Print and shaded views of the part. All mm, measured from the part's lowest x, y and z. A direction names the side the tool comes from. Give positions to 0.01 mm unless a question says otherwise; leave off trailing zeros. Write each loop counter-clockwise with the first axis right and the second up, starting at its lowest first coordinate (ties: lowest second). Pieces come first, ordered by that corner, then holes. Notation, with made-up numbers: M 21.5,27.5 L 55.5,27.5 A22 ccw 55.5,47.5 Z; hole C -10,41 d7. An arc over 180 degrees is marked long. One line per question, with ' | ' between items. Start each with the question number.
1. Wall check: L1, parallel to X at y = 2.8, z = 6.7 (3 decimals); L2, parallel to X at y = 6.75, z = 4.25; L3, parallel to Y at x = 12.5, z = 8. Give the ranges that are in metal, low to high.
2. Cut at C-C, the plane x = 10.25. Write the cut outline in (y, z), then the cut area to 3 significant figures.
3. Which spindle directions (+Z, -Z, +X, -X, +Y, -Y) get a long thin tool onto all of the face, cutting with end or side? Do the marked faces 1 and 2. Say none if no direction does.
4. Pull direction X, two halves, no side cores. Call the marked faces 3, 4, 5 and 6: released by +X, released by -X, zero draft, split by the parting line, or undercut.
5. Cut at D-D, the plane z = 9.25. Write the cut outline in (x, y), then the cut area to 3 significant figures.
6. Cut at B-B, the plane y = 1.75. Write the cut outline in (x, z) (3 decimals).
7. Cut at A-A, the plane z = 6.7. Write the cut outline in (x, y) (3 decimals), then the cut area to 4 significant figures.
8. Flat gauge pin, fed straight in: pin 1 (6 mm diameter, centred on x = 9.225, z = 6.7, fed in from +Y). Where does the tip first touch, or does it go through?
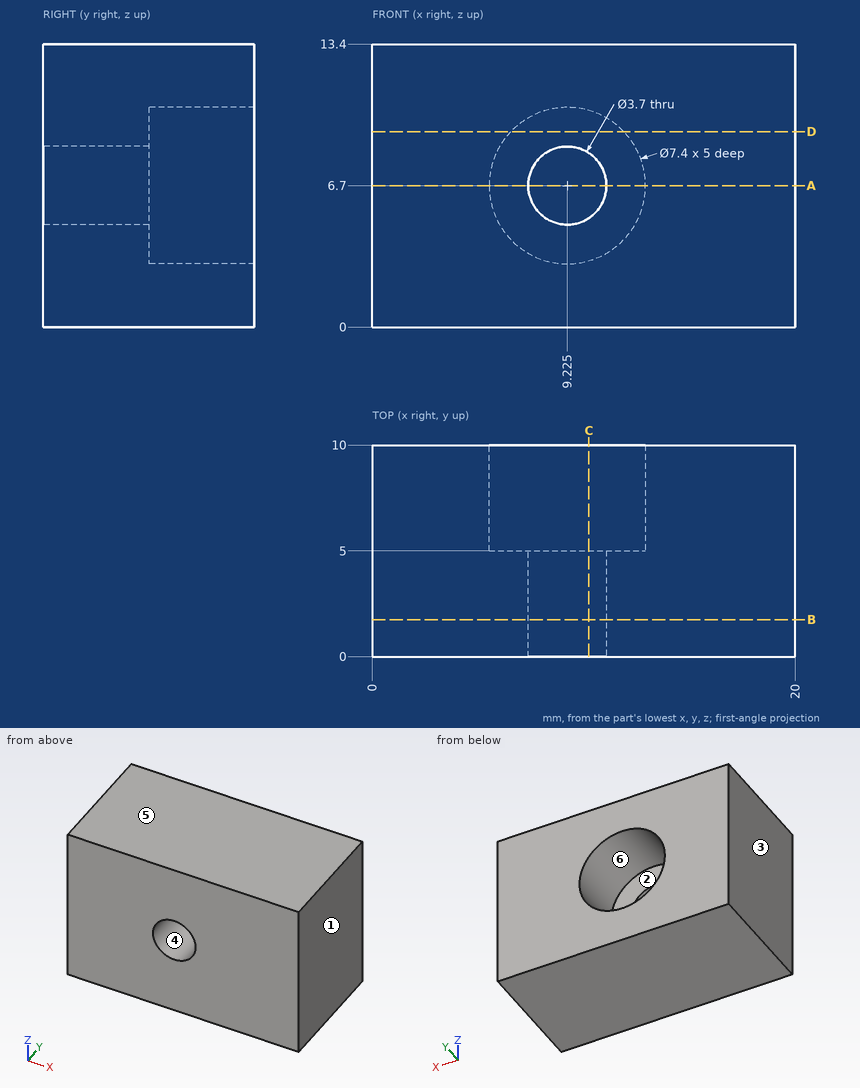
Here are the results:
1) L1: 0 to 7.375, 11.075 to 20 | L2: 0 to 6.45, 12 to 20 | L3: 0 to 5
2) outline: M 0,0 L 10,0 L 10,3.14 L 5,3.14 L 5,5.16 L 0,5.16 Z; M 0,8.24 L 5,8.24 L 5,10.26 L 10,10.26 L 10,13.4 L 0,13.4 Z | area: 83.0 mm^2
3) face 1: +Z, -Z, +X, +Y, -Y | face 2: +Y
4) face 3: released by -X | face 4: undercut | face 5: zero draft | face 6: undercut
5) outline: M 0,0 L 20,0 L 20,10 L 11.91,10 L 11.91,5 L 6.54,5 L 6.54,10 L 0,10 Z | area: 173 mm^2
6) outline: M 0,0 L 20,0 L 20,13.4 L 0,13.4 Z; hole C 9.225,6.7 d3.7
7) outline: M 0,0 L 7.375,0 L 7.375,5 L 5.525,5 L 5.525,10 L 0,10 Z; M 11.075,0 L 20,0 L 20,10 L 12.925,10 L 12.925,5 L 11.075,5 Z | area: 144.5 mm^2
8) pin 1: y = 5
